Answer from the drawing. Dimensions are ordinates in mm from the lowest x, y and z of the part. A direction names the side the tool comes from. Round coordinates to 2 decimals unless told otherwise and drop trailing zeros. Write each loop counter-clockwise with the first axis right and the second up, starting at its lowest first coordinate (ties: lowest second). Pieces come first, ordered by that corner, then holes.
1. Find section C-C (y = 50.8). Write down the section's boundary in (x, z).
2. A tool of negligible diameter and unlimited length cuts with its end or side. For the marked faces 1, 2 and 3, from which of +Z, -Z, +X, -X, +Y, -Y can it reach the whole face along a straight path? Write none if from no direction.
3. Determine the mould class of the marked faces 4, 5, 6 and 7 for opening direction Y: pulls with the +Y half, pulls with the -Y half, needs draft (parallel to the pull), parting line crosses it, or undercut.
4. Find section D-D (x = 54). Write down the section's boundary in (y, z), and give its area (3 significant figures).
5. Find section B-B (x = 38.5). Write down the section's boundary in (y, z), and give its area (3 significant figures).
6. Find section A-A (z = 14.5). Write down the section's boundary in (x, y), and give its area (3 significant figures).
7. Straight lines are drawn through the part: probe 1 along Y at (x, z) = (38.1, 55); probe 2 along Y at (x, z) = (38.1, 32); probe 3 along X at (y, z) = (50, 49). For each, find the intervals that lie inside material, in ascending order.
8. Flat-ended cylindrical pins translate along their axes: pin 1 Ø10 at (x, y) = (34, 6) entering from -Z; pin 2 Ø3 at (y, z) = (33.5, 49) entering from +X; pin 3 Ø6.5 at (y, z) = (5.5, 34.5) entering from +X; pin 4 Ø20.5 at (x, y) = (38.1, 50.8) entering from +Z. Find the tip coordinate at first contact, or state that the pin passes through.
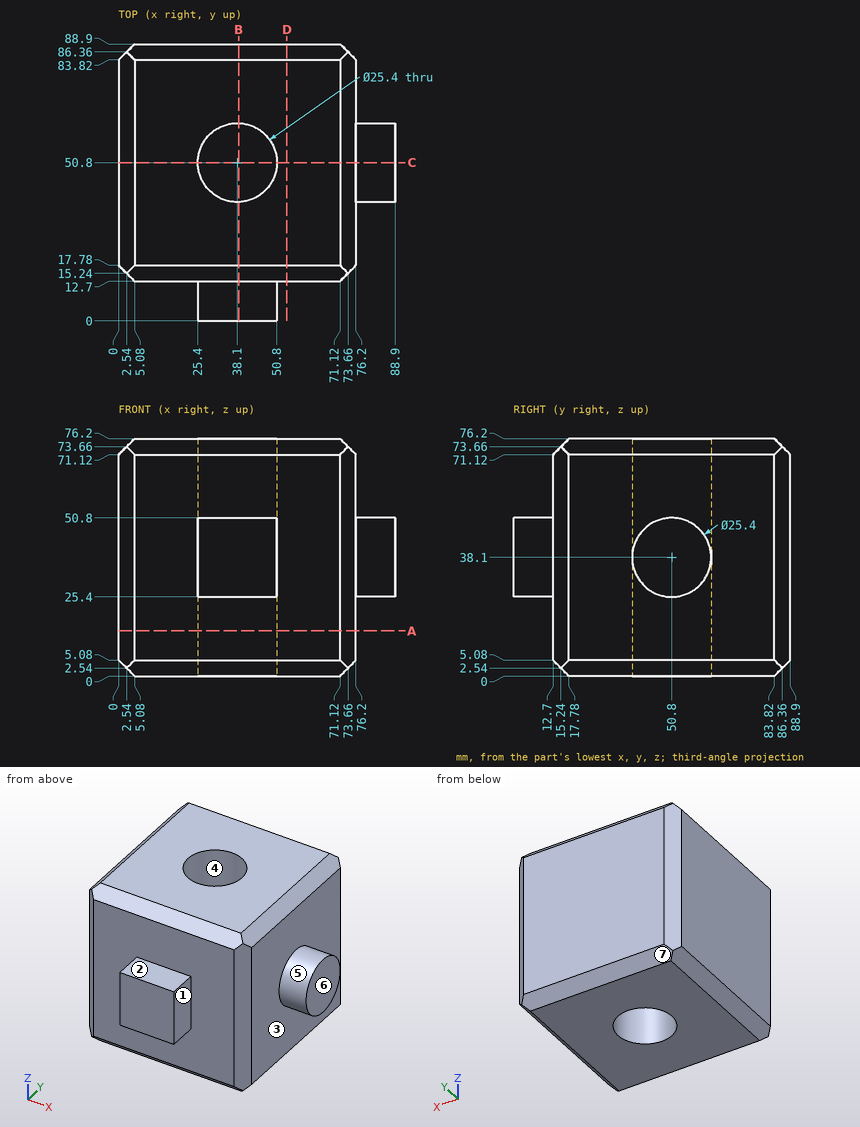
Worked answers:
1. outline: (0, 5.08) - (5.08, 0) - (25.4, 0) - (25.4, 76.2) - (5.08, 76.2) - (0, 71.12) - close; (50.8, 0) - (71.12, 0) - (76.2, 5.08) - (76.2, 25.4) - (88.9, 25.4) - (88.9, 50.8) - (76.2, 50.8) - (76.2, 71.12) - (71.12, 76.2) - (50.8, 76.2) - close
2. face 1: +Z, -Z, +X, -Y
2. face 2: +Z, +X, -X, -Y
2. face 3: +X
3. face 4: undercut
3. face 5: parting line crosses it
3. face 6: needs draft
3. face 7: pulls with the +Y half
4. outline: (12.7, 5.08) - (17.78, 0) - (83.82, 0) - (88.9, 5.08) - (88.9, 71.12) - (83.82, 76.2) - (17.78, 76.2) - (12.7, 71.12) - close
4. area: 5,750 mm2
5. outline: (0, 25.4) - (12.7, 25.4) - (12.7, 5.08) - (17.78, 0) - (38.11, 0) - (38.11, 76.2) - (17.78, 76.2) - (12.7, 71.12) - (12.7, 50.8) - (0, 50.8) - close; (63.49, 0) - (83.82, 0) - (88.9, 5.08) - (88.9, 71.12) - (83.82, 76.2) - (63.49, 76.2) - close
5. area: 4,140 mm2
6. outline: (0, 17.78) - (5.08, 12.7) - (71.12, 12.7) - (76.2, 17.78) - (76.2, 83.82) - (71.12, 88.9) - (5.08, 88.9) - (0, 83.82) - close; hole circle Ø25.4 at (38.1, 50.8)
6. area: 5,250 mm2
7. probe 1: y = 12.7 to 38.1, 63.5 to 88.9
7. probe 2: y = 0 to 38.1, 63.5 to 88.9
7. probe 3: x = 0 to 25.43, 50.77 to 88.9
8. pin 1: stops at z = 25.4
8. pin 2: stops at x = 76.2
8. pin 3: stops at x = 50.8
8. pin 4: passes through
